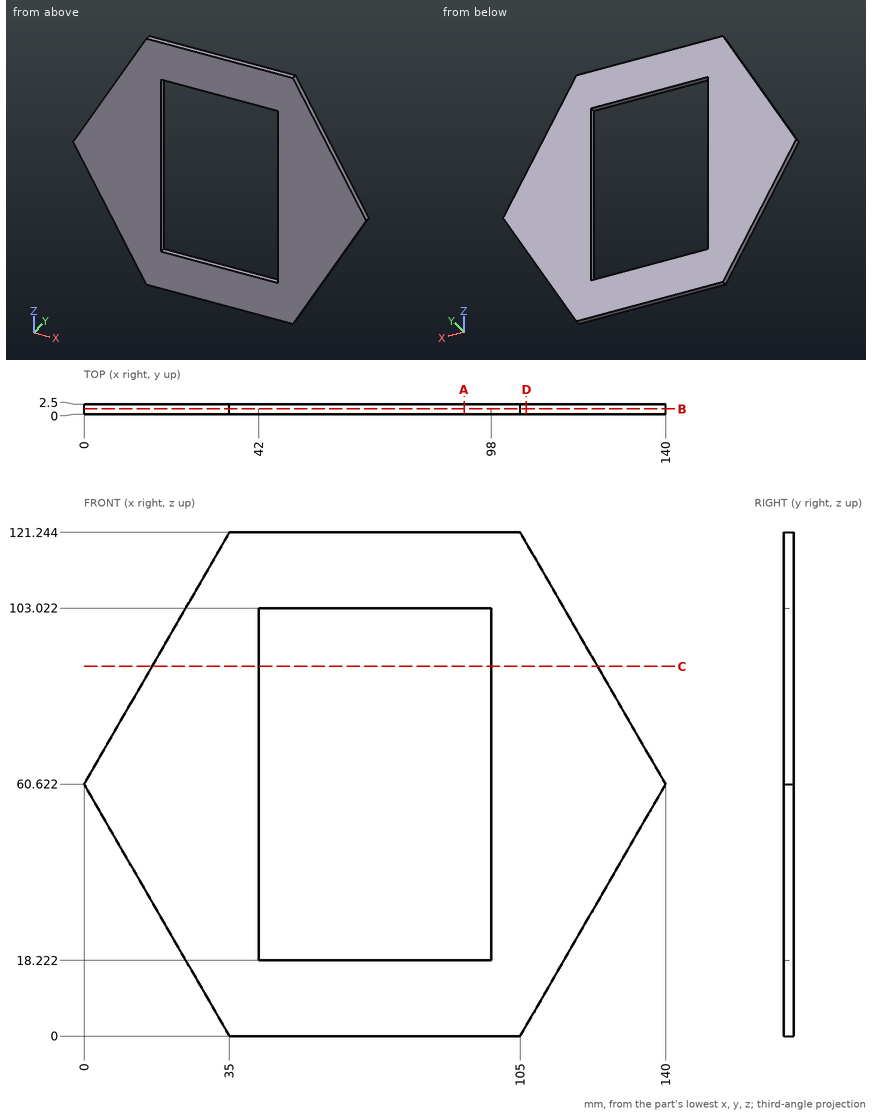
Geometry: see drawing. Coordinates: mm, zero at the bounding-box minimum. Give positions to 0.01 mm unless a question says otherwise; leave off trailing zeros. Loops run counter-clockwise (first coordinate to the right, second up) from the corner with the lowest first, then second, coordinate; pieces in that order, holes last. Notation, with made-up numbers: (28, 62) - (50, 62) arc R16 ccw to (50, 69) - close; hole circle Ø9 at (53, 10.5). An arc over 180 degrees is marked (long way). Use CSV: the item, a comma, the result in double quotes.
1) Cut plane D-D (x = 106.5). Output: boundary loops of the cut face in (y, z) (1 decimal), and give its area (3 significant figures).
Worked out:
outline,"(0, 2.6) - (2.5, 2.6) - (2.5, 118.6) - (0, 118.6) - close"
area,"290 mm^2"
2) Cut plane C-C (z = 89). Output: boundary loops of the cut face in (x, y).
Worked out:
outline,"(16.38, 0) - (42, 0) - (42, 2.5) - (16.38, 2.5) - close; (98, 0) - (123.62, 0) - (123.62, 2.5) - (98, 2.5) - close"
3) Pin query (flat end, axial travel): P1, Ø1.2, axis at y = 1.5, z = 40.5, coming from the +X side; P2, Ø1.5, axis at y = 1, z = 100, coming from the +X side. Return the tip coordinate at first contact, or that it passes through.
Worked out:
P1,"stops at x = 128.73"
P2,"stops at x = 117.7"
4) Line query: line 1 (Z direction, x = 73.5, y = 0.9); line 2 (X direction, y = 1.1, z = 91.5); line 3 (X direction, y = 0.4, z = 46.5). Output: solid intervals per line, ascending.
Worked out:
line 1,"z = 0 to 18.22, 103.02 to 121.24"
line 2,"x = 17.83 to 42, 98 to 122.17"
line 3,"x = 8.15 to 42, 98 to 131.85"
5) Cut plane B-B (y = 1.35). Output: boundary loops of the cut face in (x, z), and give its area (3 significant figures).
Worked out:
outline,"(0, 60.62) - (35, 0) - (105, 0) - (140, 60.62) - (105, 121.24) - (35, 121.24) - close; hole (42, 18.22) - (98, 18.22) - (98, 103.02) - (42, 103.02) - close"
area,"7,980 mm^2"
6) Cut plane A-A (x = 91.5). Output: boundary loops of the cut face in (y, z).
Worked out:
outline,"(0, 0) - (2.5, 0) - (2.5, 18.22) - (0, 18.22) - close; (0, 103.02) - (2.5, 103.02) - (2.5, 121.24) - (0, 121.24) - close"
